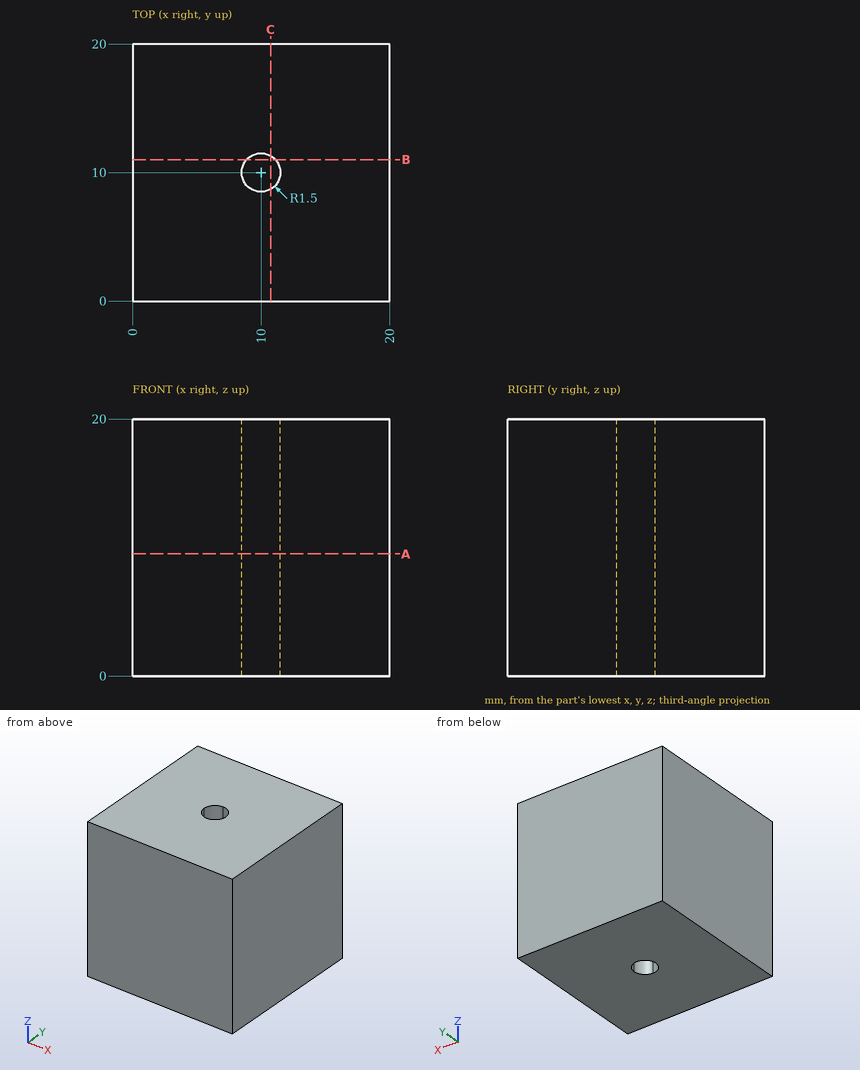
Geometry: see drawing. Coordinates: mm, zero at the bounding-box minimum. Give positions to 0.01 mm unless a question says otherwise; leave off trailing zeros. Loops run counter-clockwise (first coordinate to the right, second up) from the corner with the lowest first, then second, coordinate; pieces in that order, holes last. Notation, with made-up numbers: (-34.75, -1.5) -> (-10.75, -1.5) arc R25 cw to (-10.75, 37.5) -> close; hole circle Ø1 at (-22.5, -10). An arc over 180 degrees is marked (long way). Put each result on its own line as item: value.
1. Cut plane B-B (y = 11). Return the cut outline in (x, z).
Taken from the geometry:
outline: (0, 0) -> (8.88, 0) -> (8.88, 20) -> (0, 20) -> close; (11.12, 0) -> (20, 0) -> (20, 20) -> (11.12, 20) -> close
2. Ray query, line 1 along Y through (x, z) = (11.25, 10); line 2 along Y through (x, z) = (11, 14.5); line 3 along X through (y, z) = (9.75, 8). Return the intervals inside material, ascending. Write a range as [from, to].
Taken from the geometry:
line 1: y = [0, 9.17], [10.83, 20]
line 2: y = [0, 8.88], [11.12, 20]
line 3: x = [0, 8.52], [11.48, 20]
3. Cut plane C-C (x = 10.75). Return the cut outline in (y, z).
Taken from the geometry:
outline: (0, 0) -> (8.7, 0) -> (8.7, 20) -> (0, 20) -> close; (11.3, 0) -> (20, 0) -> (20, 20) -> (11.3, 20) -> close
4. Cut plane A-A (z = 9.5). Return the cut outline in (x, y).
Taken from the geometry:
outline: (0, 0) -> (20, 0) -> (20, 20) -> (0, 20) -> close; hole (8.5, 10) arc R1.5 ccw to (10, 8.5) arc R1.5 ccw to (11.5, 10) arc R1.5 ccw to (10, 11.5) arc R1.5 ccw to start
